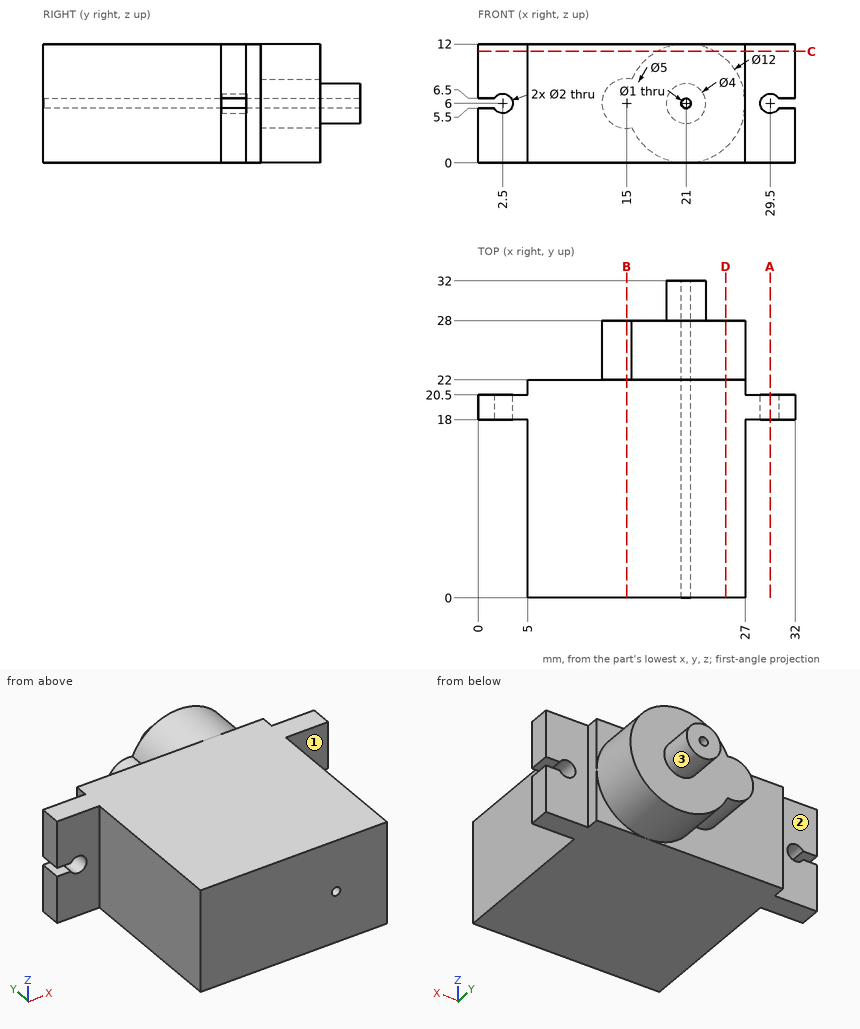
Design review of the part shown in the three views and the two pictorial views. Dimensions are in mm from the part's minimum x, y and z. A direction names the side the tool comes from. Round coordinates to 2 decimals unless told otherwise and drop trailing zeros. Write each loop counter-clockwise with the first axis right and the second up, starting at its lowest first coordinate (ties: lowest second). Pieces come first, ordered by that corner, then holes. Notation, with made-up numbers: M -37,87 L 8,87 A21 ccw 8,110 Z; hole C 40.25,-10 d10. An arc over 180 degrees is marked long. One line per item, written item: value. Start each with the question number.
1. Take a section at D-D on x = 25. State the section outline as (y, z) points, then the cut area to 3 significant figures.
2. Clearance check with flat-ended pins moving along their axes: P1, Ø5.5, axis at x = 28.5, z = 9, coming from the +Y side; P2, Ø1.8, axis at x = 29.5, z = 6, coming from the -Y side; P3, Ø2.5, axis at x = 3, z = 5.5, coming from the -Y side; P4, Ø4, axis at y = 25, z = 5, coming from the +X side. State where each tip first meets the part, or that it passes through.
3. To check wall thickness, follow probe 1 along Z at (x, y) = (21, 12.5); probe 2 along X at (y, z) = (19, 6); probe 3 along X at (y, z) = (9, 6). State the ranges of each line that lie inside material, in increasing order. Write a range as from..to.
4. For the marked faces 1, 2 and 3, list the 3-axis set-ups (+Z, -Z, +X, -X, +Y, -Y) from which the entire face can be reached by the end or side of a thin tool; tool diameter is ignored.
5. Take a section at A-A on x = 29.5. State the section outline as (y, z) points.
6. Take a section at B-B on x = 15. State the section outline as (y, z) points, then the cut area to 3 significant figures.
7. Take a section at C-C on z = 11.25. State the section outline as (x, y) points.
Computed:
1. outline: M 0,0 L 22,0 L 22,1.53 L 28,1.53 L 28,10.47 L 22,10.47 L 22,12 L 0,12 Z
1. area: 318 mm²
2. P1: stops at y = 28
2. P2: passes through
2. P3: stops at y = 18
2. P4: stops at x = 27
3. probe 1: z = 0..5.5, 6.5..12
3. probe 2: x = 3.5..20.5, 21.5..28.5
3. probe 3: x = 5..20.5, 21.5..27
4. face 1: +Z, -Z, +X, -Y
4. face 2: +Z, -Z, -X, +Y
4. face 3: +Y
5. outline: M 18,0 L 20.5,0 L 20.5,5 L 18,5 Z; M 18,7 L 20.5,7 L 20.5,12 L 18,12 Z
6. outline: M 0,0 L 22,0 L 22,3.5 L 28,3.5 L 28,8.5 L 22,8.5 L 22,12 L 0,12 Z
6. area: 294 mm²
7. outline: M 0,18 L 5,18 L 5,0 L 27,0 L 27,18 L 32,18 L 32,20.5 L 27,20.5 L 27,22 L 23.9,22 L 23.9,28 L 18.1,28 L 18.1,22 L 5,22 L 5,20.5 L 0,20.5 Z
